```python
from build123d import *

# Parameters (mm, degrees)
F0_W     = 38.1
F0_H     = 50.8
F0_W_2   = 25.4
F0_H_2   = 12.7
F1_DEPTH = 35.052
F2_R     = 5.08


with BuildPart() as f1:
    # F0 (on Top) → F1 (new body)
    with BuildSketch(Plane.XY):
        with Locations((5.208455, 14.55895)):
            Rectangle(F0_W, F0_H)
        with Locations((-26.541545, -17.19105)):
            Rectangle(F0_W_2, F0_H_2)
        with Locations((5.208455, -17.19105)):
            Rectangle(F0_W, F0_H_2)
        with Locations((36.958455, -17.19105)):
            Rectangle(F0_W_2, F0_H_2)
    extrude(amount=F1_DEPTH)

    # F2
    f2_edges = [f1.edges().sort_by_distance(p)[0] for p in [
        (24.258455, 14.55895, 35.052),
        (-13.841545, 14.55895, 35.052),
        (-26.541545, -10.84105, 35.052),
        (36.958455, -10.84105, 35.052),
        (5.208455, -23.54105, 35.052),
    ]]
    fillet(f2_edges, radius=F2_R)


solid = f1.part
```
CAD build for the part. Positions are in the model's coordinates, mm. A direction names the side the tool comes from. Coordinates: 2 decimals unless noted, no trailing zeros. Order: outer loops, then holes, each group sorted by start corner. A loop starts at its lowest first (then second) coordinate and runs counter-clockwise, first axis right, second up. Notation, with made-up numbers: (33.5, 58.5) -> (77.5, 58.5) arc R16 ccw to (77.5, 84.5) -> close; hole circle Ø7 at (19, 15.5). An arc over 180 degrees is marked (long way). Use one line per item in the form item = value. Start each with the question number.
1) Band-saw the part on C-C on z = 31. Give the cut face in (x, y).
2) Band-saw the part on A-A on z = 15. Give the cut face in (x, y), then the cut area to 3 significant figures.
3) Band-saw the part on B-B on y = -0.5. Give the cut face in (x, z).
4) Tool access for faces 1 (the cylindrical face through (22.81, 12.41, 33.524)), 2 (the flat face through (24.258, 14, 15)), 3 (the flat face through (-13.842, 14, 15)): list every direction of +Z, -Z, +X, -X, +Y, -Y with a clear straight run to the whole face (end or side of a thin tool).
5) Drill centre lines: L1, parallel to X at y = 5, z = 25.5; L2, parallel to Y at x = 33.5, z = 18.5; L3, parallel to X at y = 28.5, z = 31.5. Where is each one in solid material? Low to high. Write a range as [from, to].
6) Drop flat-ended pins along their axis: pin 1 (6 mm diameter, centred on y = 9.5, z = 5.5, fed in from -X); pin 2 (4 mm diameter, centred on x = 17.5, y = -10.5, fed in from -Z); pin 3 (12 mm diameter, centred on y = 30, z = 17.5, fed in from +X). Give the stop position or say it passes through.
Entries:
q1.outline = (-39.24, -23.44) -> (49.66, -23.44) -> (49.66, -10.95) -> (24.15, -10.95) -> (24.15, 39.96) -> (-13.74, 39.96) -> (-13.74, -10.95) -> (-39.24, -10.95) -> close
q2.outline = (-39.24, -23.54) -> (49.66, -23.54) -> (49.66, -10.84) -> (24.26, -10.84) -> (24.26, 39.96) -> (-13.84, 39.96) -> (-13.84, -10.84) -> (-39.24, -10.84) -> close
q2.area = 3,060 mm2
q3.outline = (-13.84, 0) -> (24.26, 0) -> (24.26, 29.97) arc R5.08 ccw to (19.18, 35.05) -> (-8.76, 35.05) arc R5.08 ccw to (-13.84, 29.97) -> close
q4.face_1 = +Z, +X, +Y
q4.face_2 = +Z, -Z, +X, +Y
q4.face_3 = +Z, -Z, -X, +Y
q5.L1 = [-13.84, 24.26]
q5.L2 = [-23.54, -10.84]
q5.L3 = [-13.61, 24.02]
q6.pin_1 = -13.84
q6.pin_2 = 0
q6.pin_3 = 24.26
